from build123d import *

# Parameters (mm, degrees)
SKETCH1_W               = 1000
SKETCH1_H               = 1000
BOSS_EXTRUDE1_DEPTH     = 150
SKETCH2_R               = 300
CUT_EXTRUDE1_DEPTH      = 100
FILLET1_R               = 20
SKETCH3_R               = 10
CUT_EXTRUDE2_DEPTH      = 100
MIRROR2_COPY_1_SKETCH_R = 10
MIRROR2_COPY_1_DEPTH    = 100


with BuildPart() as part:
    # Sketch1 → Boss-Extrude1 (new body)
    with BuildSketch(Plane(origin=(0, 0, 0), x_dir=(1, 0, 0), z_dir=(0, 1, 0))):
        Rectangle(SKETCH1_W, SKETCH1_H)
    extrude(amount=BOSS_EXTRUDE1_DEPTH)

    # Sketch2 → Cut-Extrude1 (cut)
    with BuildSketch(Plane.XZ):
        Circle(SKETCH2_R)
    extrude(amount=-CUT_EXTRUDE1_DEPTH, mode=Mode.SUBTRACT)

    # Fillet1
    fillet1_edges = [part.edges().sort_by_distance(p)[0] for p in [
        (500, 150, 0),
        (0, 150, -500),
        (-500, 150, 0),
        (-500, 75, -500),
        (500, 75, -500),
        (500, 75, 500),
        (-500, 75, 500),
        (0, 150, 500),
    ]]
    fillet(fillet1_edges, radius=FILLET1_R)

    # Sketch3 → Cut-Extrude2 (cut)
    with BuildSketch(Plane.XZ):
        with Locations((-460, -400)):
            Circle(SKETCH3_R)
    cut_extrude2 = extrude(amount=-CUT_EXTRUDE2_DEPTH, mode=Mode.SUBTRACT)

    # Mirror1: Cut-Extrude2 across plane
    add(cut_extrude2.mirror(Plane(origin=(0, 0, 0), x_dir=(0, 0, 1), z_dir=(1, 0, 0))), mode=Mode.SUBTRACT)

    # Mirror2: Cut-Extrude2 across plane
    add(cut_extrude2.mirror(Plane.XY), mode=Mode.SUBTRACT)

    # Mirror2 copy 1 sketch → Mirror2 copy 1 (cut)
    with BuildSketch(Plane(origin=(0, 0, 0), x_dir=(-1, 0, 0), z_dir=(0, -1, 0))):
        with Locations((-460, -400)):
            Circle(MIRROR2_COPY_1_SKETCH_R)
    extrude(amount=-MIRROR2_COPY_1_DEPTH, mode=Mode.SUBTRACT)


solid = part.part
Design review of the part built by this model. Coordinates are the model's own, in mm. A direction names the side the tool comes from. Round coordinates to 2 decimals unless told otherwise and drop trailing zeros. Write each loop counter-clockwise with the first axis right and the second up, starting at its lowest first coordinate (ties: lowest second). Pieces come first, ordered by that corner, then holes. Notation, with made-up numbers: (70, 16) -> (86, 16) arc R19 ccw to (86, 36) -> close; hole circle Ø7 at (45.5, -2). An arc over 180 degrees is marked (long way). One line per item, written item: value. Start each with the question number.
Q1. Tool access review of faces 1 (the face through (-4, 100, 4)), 2 (the face through (-229, 0, -229)): name each direction out of +Z, -Z, +X, -X, +Y, -Y from which nothing blocks a thin tool from reaching the whole face with its end or side.
Q2. Add section B-B (y = 79). Give the boundary of the cut face in (x, z), then the cut area to 3 significant figures.
Q3. To check wall thickness, follow probe 1 along Z at (x, y) = (460, 53); probe 2 along X at (y, z) = (35, 400); probe 3 along Z at (x, y) = (9, 26). State the ranges of each line that lie inside material, in increasing order.
Q4. Add section C-C (z = 0). Give the boundary of the cut face in (x, y).
Q5. Add section A-A (x = 0). Give the boundary of the cut face in (y, z), then the cut area to 3 significant figures.
Q6. The part is to be moulded in two halves that separate along X. For faces 3 (the face through (-39.054, 49.3, 297.447)), 4 (the face through (500, 64, 7)), 5 (the face through (-7, 64, 500)), say which applies: pulls with the +X half, pulls with the -X half, needs draft (parallel to the pull), parting line crosses it, or undercut.
Q7. Insertion check: P1, Ø6, axis at x = 461.5, z = 402, coming from the -Y side. The pin has a flat end and moves straight along its axis. Give the tip position at first contact, or say it passes through.
Response:
1. face 1: -Y
1. face 2: +Z, -Z, +X, -X, -Y
2. outline: (-500, -480) arc R20 ccw to (-480, -500) -> (480, -500) arc R20 ccw to (500, -480) -> (500, 480) arc R20 ccw to (480, 500) -> (-480, 500) arc R20 ccw to (-500, 480) -> close; hole circle Ø20 at (-460, -400); hole circle Ø20 at (-460, 400); hole circle Ø600 at (0, 0); hole circle Ø20 at (460, -400); hole circle Ø20 at (460, 400)
2. area: 716,000 mm^2
3. probe 1: z = -500 to -410, -390 to 390, 410 to 500
3. probe 2: x = -500 to -470, -450 to 450, 470 to 500
3. probe 3: z = -500 to -299.86, 299.86 to 500
4. outline: (-500, 0) -> (-300, 0) -> (-300, 100) -> (300, 100) -> (300, 0) -> (500, 0) -> (500, 130) arc R20 ccw to (480, 150) -> (-480, 150) arc R20 ccw to (-500, 130) -> close
5. outline: (0, -500) -> (130, -500) arc R20 ccw to (150, -480) -> (150, 480) arc R20 ccw to (130, 500) -> (0, 500) -> (0, 300) -> (100, 300) -> (100, -300) -> (0, -300) -> close
5. area: 89,800 mm^2
6. face 3: undercut
6. face 4: pulls with the +X half
6. face 5: needs draft
7. P1: stops at y = 100
